The figure shows three views and two pictorial views of one solid part (mm, origin at its lowest corner). Answer the questions. A direction names the side the tool comes from. Give positions to 0.01 mm unless a question says otherwise; leave off trailing zeros. Loops run counter-clockwise (first coordinate to the right, second up) from the corner with the lowest first, then second, coordinate; pieces in that order, holes last. Notation, with made-up numbers: M -9.5,68 L 10.5,68 A31 ccw 10.5,96 Z; hole C -39.5,-24.5 d1. An arc over 180 degrees is marked long. One line per item, written item: value. Start each with the question number.
Q1. For the marked faces 4, 5 and 6, determine the directions among +Z, -Z, +X, -X, +Y, -Y from which every point of the face is accessible in a straight line to the end or side of a thin tool.
Q2. Flat-ended cylindrical pins translate along their axes: pin 1 (2 mm diameter, centred on x = 10, y = 8.5, fed in from +Z); pin 2 (1.9 mm diameter, centred on y = 2.5, z = 2.5, fed in from -X) (3 decimals); pin 3 (0.5 mm diameter, centred on x = 7, z = 2.5, fed in from -Y). Find the tip coordinate at first contact, or state that the pin passes through.
Q3. A cutting plane is placed at B-B, the plane z = 2. Determine the outline of the cut face in (x, y) (3 decimals), and give its area (3 significant figures).
Q4. A cutting plane is placed at A-A, the plane y = 3.75. Determine the outline of the cut face in (x, z) (3 decimals), and give its area (3 significant figures).
Q5. A cutting plane is placed at C-C, the plane y = 12.5. Determine the outline of the cut face in (x, z) (3 decimals).
Q6. A cutting plane is placed at D-D, the plane x = 17.75. Determine the outline of the cut face in (y, z).
Q7. Consider L1, parallel to X at y = 4, z = 0.5 (3 decimals); L2, parallel to X at y = 11.75, z = 6.25 (3 decimals); L3, parallel to Y at x = 8, z = 2.75. Determine where each line is inside the solid, lowest interval first.
Q8. The mould has two halves that part along X. Classify the marked faces 1, 2 and 3: +X half, -X half, draft (parallel to the pull), parting line (faces both ways), or undercut.
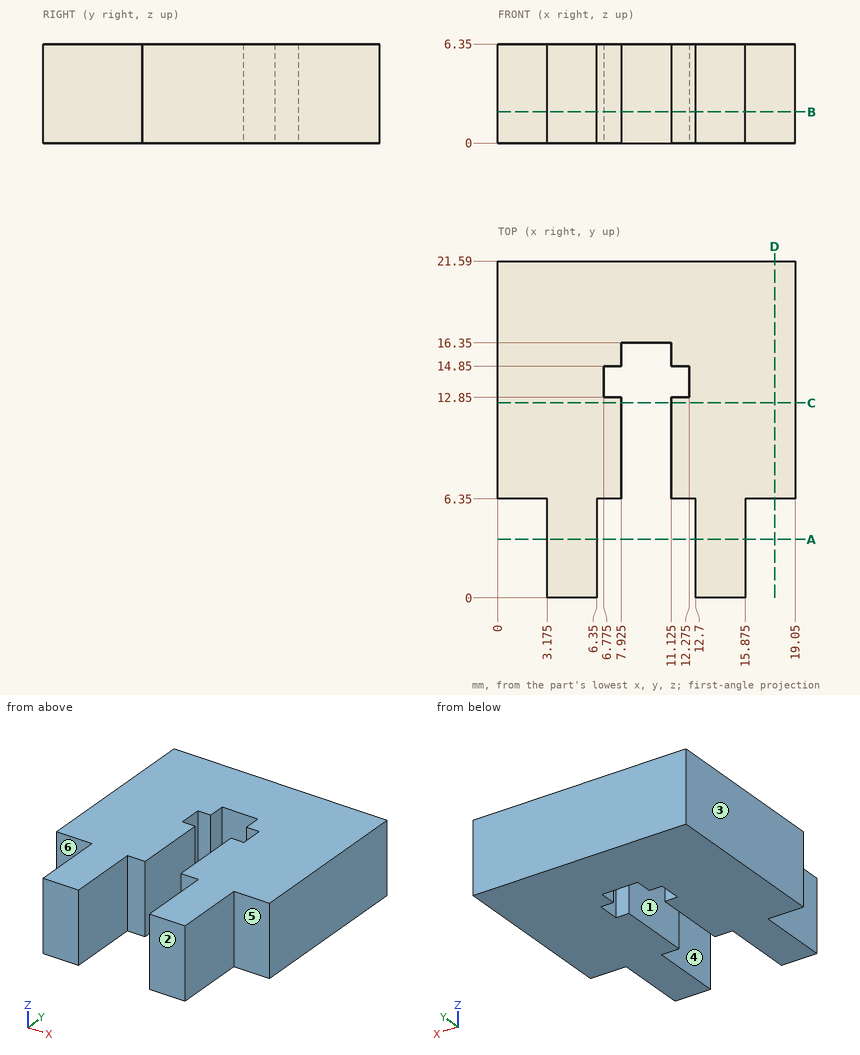
Answer block:
1. face 4: +Z, -Z, -Y
1. face 5: +Z, -Z, +X, -Y
1. face 6: +Z, -Z, -X, -Y
2. pin 1: through
2. pin 2: x = 3.175
2. pin 3: y = 6.35
3. outline: M 0,6.35 L 3.175,6.35 L 3.175,0 L 6.35,0 L 6.35,6.35 L 7.925,6.35 L 7.925,12.85 L 6.775,12.85 L 6.775,14.85 L 7.925,14.85 L 7.925,16.35 L 11.125,16.35 L 11.125,14.85 L 12.275,14.85 L 12.275,12.85 L 11.125,12.85 L 11.125,6.35 L 12.7,6.35 L 12.7,0 L 15.875,0 L 15.875,6.35 L 19.05,6.35 L 19.05,21.59 L 0,21.59 Z
3. area: 294 mm^2
4. outline: M 3.175,0 L 6.35,0 L 6.35,6.35 L 3.175,6.35 Z; M 12.7,0 L 15.875,0 L 15.875,6.35 L 12.7,6.35 Z
4. area: 40.3 mm^2
5. outline: M 0,0 L 7.925,0 L 7.925,6.35 L 0,6.35 Z; M 11.125,0 L 19.05,0 L 19.05,6.35 L 11.125,6.35 Z
6. outline: M 6.35,0 L 21.59,0 L 21.59,6.35 L 6.35,6.35 Z
7. L1: 3.175 to 6.35, 12.7 to 15.875
7. L2: 0 to 7.925, 11.125 to 19.05
7. L3: 16.35 to 21.59
8. face 1: undercut
8. face 2: draft
8. face 3: -X half
